from build123d import *

# Parameters (mm, degrees)
SKETCH2_W           = 100
SKETCH2_H           = 110
SKETCH2_R           = 1.25
BOSS_EXTRUDE1_DEPTH = 2
SKETCH3_W           = 15
SKETCH3_H           = 20
SKETCH3_W_2         = 6
BOSS_EXTRUDE2_DEPTH = 20


with BuildPart() as part:
    # Sketch2 → Boss-Extrude1 (new body)
    with BuildSketch(Plane(origin=(0, 0, 0), x_dir=(1, 0, 0), z_dir=(0, 1, 0))):
        Rectangle(SKETCH2_W, SKETCH2_H)
        with Locations((-45, 50.25)):
            Circle(SKETCH2_R, mode=Mode.SUBTRACT)
        with Locations((45, 50.25)):
            Circle(SKETCH2_R, mode=Mode.SUBTRACT)
        with Locations((45, -50.25)):
            Circle(SKETCH2_R, mode=Mode.SUBTRACT)
        with Locations((-45, -50.25)):
            Circle(SKETCH2_R, mode=Mode.SUBTRACT)
    extrude(amount=BOSS_EXTRUDE1_DEPTH)

    # Sketch3 → Boss-Extrude2 (add)
    with BuildSketch(Plane(origin=(0, 2, 0), x_dir=(1, 0, 0), z_dir=(0, 1, 0))):
        with Locations((-20, -20)):
            Rectangle(SKETCH3_W, SKETCH3_H)
        Rectangle(SKETCH3_W_2, SKETCH3_H)
        with Locations((-20, 20)):
            Rectangle(SKETCH3_W, SKETCH3_H)
        with Locations((20, 20)):
            Rectangle(SKETCH3_W, SKETCH3_H)
        with Locations((20, -20)):
            Rectangle(SKETCH3_W, SKETCH3_H)
    extrude(amount=BOSS_EXTRUDE2_DEPTH)


solid = part.part
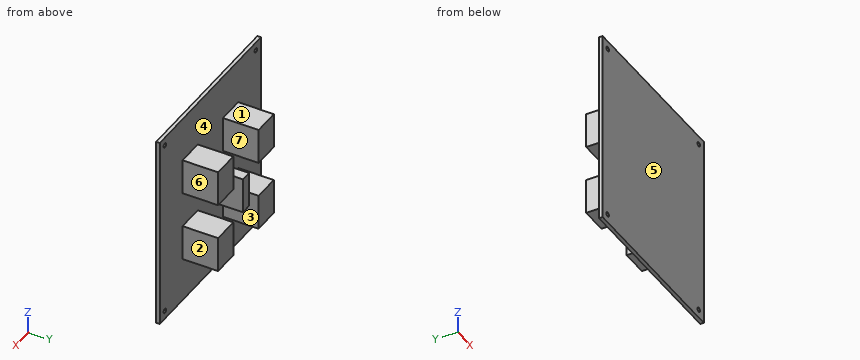
Here's how the part is built. I have some questions about the finished solid (model axes, mm). Face numbers are marked on the shaded views. A direction names the side the tool comes from. Round coordinates to 2 decimals unless told otherwise and drop trailing zeros. Loops run counter-clockwise (first coordinate to the right, second up) from the corner with the lowest first, then second, coordinate; pieces in that order, holes last. Notation, with made-up numbers: (52, -1.5) - (74, -1.5) arc R19 ccw to (74, 17.5) - close; hole circle Ø9 at (0, 70). An arc over 180 degrees is marked (long way). One line per question, with ' | ' between items. Start each with the question number.
Q1. I want a section at B-B (y = 19). Write out the boundary of the cut face in (x, z), then the cut area to 3 significant figures.
Q2. For the marked faces 1, 2 and 3, which set-ups out of +Z, -Z, +X, -X, +Y, -Y let a thin tool reach every point of the face, with its end or its side?
Q3. I want a section at A-A (x = -45). Write out the boundary of the cut face in (y, z).
Q4. We'd pull the mould along X, two halves only. Please class the marked faces 4, 5, 6 and 7: +X half, -X half, draft (parallel to the pull), parting line (faces both ways), or undercut.
Q5. Will these pins go through, and if not, where does the flat tip stop? pin 1 (10 mm diameter, centred on y = 13, z = -18, fed in from -X); pin 2 (3 mm diameter, centred on y = 5.5, z = 11, fed in from +X); pin 3 (12 mm diameter, centred on x = -30, y = 10, fed in from +Z).
Q6. Please list where these lines run through material, in increasing order: line 1 (Z direction, x = -45, y = 1.65); line 2 (X direction, y = 1.5, z = -50.25); line 3 (Z direction, x = -18.5, y = 4.25). Write a range as [from, to].
Q7. I want a section at D-D (z = 11.5). Write out the boundary of the cut face in (x, y).
Q8. I want a section at C-C (z = -50.25). Write out the boundary of the cut face in (x, y), then the cut area to 3 significant figures.
Response values:
1) outline: (-27.5, -30) - (-12.5, -30) - (-12.5, -10) - (-27.5, -10) - close; (-27.5, 10) - (-12.5, 10) - (-12.5, 30) - (-27.5, 30) - close; (-3, -10) - (3, -10) - (3, 10) - (-3, 10) - close; (12.5, -30) - (27.5, -30) - (27.5, -10) - (12.5, -10) - close; (12.5, 10) - (27.5, 10) - (27.5, 30) - (12.5, 30) - close | area: 1,320 mm²
2) face 1: +Z, +X, -X, +Y | face 2: +Z, -Z, +X, +Y | face 3: +Z, -Z, +Y
3) outline: (0, -55) - (2, -55) - (2, -51.5) - (0, -51.5) - close; (0, -49) - (2, -49) - (2, 49) - (0, 49) - close; (0, 51.5) - (2, 51.5) - (2, 55) - (0, 55) - close
4) face 4: undercut | face 5: draft | face 6: +X half | face 7: undercut
5) pin 1: stops at x = -27.5 | pin 2: stops at x = 27.5 | pin 3: stops at z = 30
6) line 1: z = [-55, -51.5], [-49, 49], [51.5, 55] | line 2: x = [-50, -46.25], [-43.75, 43.75], [46.25, 50] | line 3: z = [-30, -10], [10, 30]
7) outline: (-50, 0) - (50, 0) - (50, 2) - (27.5, 2) - (27.5, 22) - (12.5, 22) - (12.5, 2) - (-12.5, 2) - (-12.5, 22) - (-27.5, 22) - (-27.5, 2) - (-50, 2) - close
8) outline: (-50, 0) - (-46.25, 0) - (-46.25, 2) - (-50, 2) - close; (-43.75, 0) - (43.75, 0) - (43.75, 2) - (-43.75, 2) - close; (46.25, 0) - (50, 0) - (50, 2) - (46.25, 2) - close | area: 190 mm²
